Check sheet for the modelled part. Datum: model origin and axes. Units: mm. Face numbers are marked on the shaded views. A direction names the side the tool comes from. Round coordinates to 2 decimals unless told otherwise and drop trailing zeros. Loops run counter-clockwise (first coordinate to the right, second up) from the corner with the lowest first, then second, coordinate; pieces in that order, holes last. Notation, with made-up numbers: (-34.75, 45.25) -> (-18.75, 45.25) arc R8 cw to (-18.75, 56.25) -> close; hole circle Ø6 at (88, 76). An arc over 180 degrees is marked (long way). One line per question, with ' | ' between items.
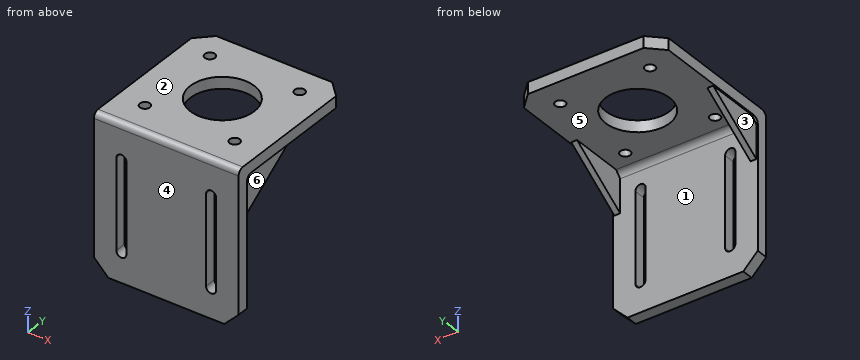
```python
from build123d import *

# Parameters (mm, degrees)
SALIENTE_EXTRUIR1_DEPTH = 50
CROQUIS2_R              = 11.05
CROQUIS2_R_2            = 1.75
CORTAR_EXTRUIR1_DEPTH   = 90.523739868
CORTAR_EXTRUIR2_DEPTH   = 90.523739868
CHAFL_N1_SIZE           = 5
SALIENTE_EXTRUIR4_DEPTH = 2
SALIENTE_EXTRUIR5_DEPTH = 2


with BuildPart() as part:
    # Croquis1 → Saliente-Extruir1 (new body)
    with BuildSketch(Plane(origin=(0, 0, 0), x_dir=(0, 0, -1), z_dir=(1, 0, 0))):
        with BuildLine():
            Line((2, 0), (53.5, 0))
            Line((53.5, 0), (53.5, 4))
            Line((53.5, 4), (6, 4))
            ThreePointArc((6, 4), (4.585786438, 4.585786438), (4, 6))
            Line((4, 6), (4, 51.5))
            Line((4, 51.5), (0, 51.5))
            Line((0, 51.5), (0, 2))
            ThreePointArc((0, 2), (0.585786438, 0.585786438), (2, 0))
        make_face()
    extrude(amount=SALIENTE_EXTRUIR1_DEPTH)

    # Croquis2 → Cortar-Extruir1 (cut, through all)
    with BuildSketch(Plane.XY):
        with Locations((25, 26.75)):
            Circle(CROQUIS2_R)
        with Locations((9.5, 42.25)):
            Circle(CROQUIS2_R_2)
        with Locations((40.5, 42.25)):
            Circle(CROQUIS2_R_2)
        with Locations((9.5, 11.25)):
            Circle(CROQUIS2_R_2)
        with Locations((40.5, 11.25)):
            Circle(CROQUIS2_R_2)
    extrude(amount=-CORTAR_EXTRUIR1_DEPTH, mode=Mode.SUBTRACT)

    # Croquis3 → Cortar-Extruir2 (cut, through all)
    with BuildSketch(Plane.XZ):
        with BuildLine():
            Line((7.75, -12.25), (7.75, -43.25))
            ThreePointArc((7.75, -43.25), (9.5, -45), (11.25, -43.25))
            Line((11.25, -43.25), (11.25, -12.25))
            ThreePointArc((11.25, -12.25), (9.5, -10.5), (7.75, -12.25))
        make_face()
        with BuildLine():
            Line((38.75, -12.25), (38.75, -43.25))
            ThreePointArc((38.75, -43.25), (40.5, -45), (42.25, -43.25))
            Line((42.25, -43.25), (42.25, -12.25))
            ThreePointArc((42.25, -12.25), (40.5, -10.5), (38.75, -12.25))
        make_face()
    extrude(amount=-CORTAR_EXTRUIR2_DEPTH, mode=Mode.SUBTRACT)

    # Chaflán1
    chafl_n1_edges = [part.edges().sort_by_distance(p)[0] for p in [
        (0, 2, -53.5),
        (50, 51.5, -2),
        (50, 2, -53.5),
        (0, 51.5, -2),
    ]]
    chamfer(chafl_n1_edges, length=CHAFL_N1_SIZE)

    # Croquis6 → Saliente-Extruir4 (add)
    with BuildSketch(Plane(origin=(49.5, 0, 0), x_dir=(0, 0, -1), z_dir=(1, 0, 0))):
        Polygon((4, 24.585786438), (4, 6), (6, 4), (17.585786438, 4), align=None)
    extrude(amount=-SALIENTE_EXTRUIR4_DEPTH)

    # Croquis7 → Saliente-Extruir5 (add)
    with BuildSketch(Plane.ZY.offset(-0.5)):
        Polygon((-17.585786438, 4), (-4, 24.585786438), (-4, 6), (-6, 4), align=None)
    extrude(amount=-SALIENTE_EXTRUIR5_DEPTH)


solid = part.part
```
(1) Sectioned sample at C-C, the plane y = 17. Record the cut outline in (x, z), and give its area (3 significant figures).
Answer:
outline: (0, -4) -> (0.5, -4) -> (0.5, -9.01) -> (2.5, -9.01) -> (2.5, -4) -> (19.8, -4) -> (19.8, 0) -> (0, 0) -> close; (30.2, -4) -> (47.5, -4) -> (47.5, -9.01) -> (49.5, -9.01) -> (49.5, -4) -> (50, -4) -> (50, 0) -> (30.2, 0) -> close | area: 178 mm2
(2) Sectioned sample at D-D, the plane x = 40.5. Record the cut outline in (y, z), and give its area (3 significant figures).
Answer:
outline: (0, -53.5) -> (4, -53.5) -> (4, -45) -> (0, -45) -> close; (0, -10.5) -> (4, -10.5) -> (4, -6) arc R2 cw to (6, -4) -> (9.5, -4) -> (9.5, 0) -> (2, 0) arc R2 ccw to (0, -2) -> close; (13, -4) -> (40.5, -4) -> (40.5, 0) -> (13, 0) -> close; (44, -4) -> (51.5, -4) -> (51.5, 0) -> (44, 0) -> close | area: 238 mm2
(3) Set-up check for the marked faces 1 and 2: record each of +Z, -Z, +X, -X, +Y, -Y from which the full face is reachable in a straight line by a thin tool's end or side.
Answer:
face 1: -Z, +Y | face 2: +Z, +X, -X, +Y, -Y
(4) Sectioned sample at B-B, the plane x = 25. Record the cut outline in (y, z).
Answer:
outline: (0, -53.5) -> (4, -53.5) -> (4, -6) arc R2 cw to (6, -4) -> (15.7, -4) -> (15.7, 0) -> (2, 0) arc R2 ccw to (0, -2) -> close; (37.8, -4) -> (51.5, -4) -> (51.5, 0) -> (37.8, 0) -> close
(5) Mould release check, pull along X, two halves, no side actions. Record for the marked faces 3, 4, 5 and 6: +X half, -X half, draft (parallel to the pull), parting line (faces both ways), or undercut.
Answer:
face 3: -X half | face 4: draft | face 5: undercut | face 6: +X half
(6) Sectioned sample at A-A, the plane z = -32. Record the cut outline in (x, y), and give its area (3 significant figures).
Answer:
outline: (0, 0) -> (7.75, 0) -> (7.75, 4) -> (0, 4) -> close; (11.25, 0) -> (38.75, 0) -> (38.75, 4) -> (11.25, 4) -> close; (42.25, 0) -> (50, 0) -> (50, 4) -> (42.25, 4) -> close | area: 172 mm2
(7) Go/stop test with flat-tipped pins: pin 1 (12 mm diameter, centred on x = 38.5, y = 40.5, fed in from -Z); pin 2 (5.5 mm diameter, centred on x = 40.5, y = 11.25, fed in from +Z); pin 3 (7 mm diameter, centred on y = 13, z = -12, fed in from +X); pin 4 (4 mm diameter, centred on y = 10, z = -9, fed in from -X). Record where each tip stops, or that it passes through.
Answer:
pin 1: stops at z = -4 | pin 2: stops at z = 0 | pin 3: stops at x = 49.5 | pin 4: stops at x = 0.5
(8) Scan lines: probe 1 along X at (y, z) = (42, -3); probe 2 along Y at (x, z) = (9.5, -3); probe 3 along Y at (x, z) = (40.5, -1.05). Record each from-to range of solid material in increasing order.
Answer:
probe 1: x = 0 to 7.77, 11.23 to 38.77, 42.23 to 50 | probe 2: y = 0 to 9.5, 13 to 40.5, 44 to 51.5 | probe 3: y = 0.24 to 9.5, 13 to 40.5, 44 to 51.5
